from build123d import *

# Parameters (mm, degrees)
SKETCH1_W           = 8.5
SKETCH1_H           = 3.65
BOSS_EXTRUDE1_DEPTH = 1
SKETCH2_W           = 2.5
SKETCH2_H           = 2.05
BOSS_EXTRUDE2_DEPTH = 3
SKETCH3_W           = 4
SKETCH3_H           = 3.65
SKETCH3_W_2         = 3
BOSS_EXTRUDE3_DEPTH = 2.2
SKETCH4_W           = 8.5
SKETCH4_H           = 1
BOSS_EXTRUDE4_DEPTH = 1


with BuildPart() as part:
    # Sketch1 → Boss-Extrude1 (new body)
    with BuildSketch(Plane.XY):
        Rectangle(SKETCH1_W, SKETCH1_H)
    extrude(amount=BOSS_EXTRUDE1_DEPTH)

    # Sketch2 → Boss-Extrude2 (add)
    with BuildSketch(Plane.XY.offset(1)):
        Rectangle(SKETCH2_W, SKETCH2_H)
    extrude(amount=BOSS_EXTRUDE2_DEPTH)

    # Sketch3 → Boss-Extrude3 (add)
    with BuildSketch(Plane(origin=(0, 0, 0), x_dir=(-1, 0, 0), z_dir=(0, 0, -1))):
        with Locations((2.25, 0)):
            Rectangle(SKETCH3_W, SKETCH3_H)
        with Locations((-2.75, 0)):
            Rectangle(SKETCH3_W_2, SKETCH3_H)
    extrude(amount=BOSS_EXTRUDE3_DEPTH)

    # Sketch4 → Boss-Extrude4 (add)
    with BuildSketch(Plane(origin=(0, 1.825, 0), x_dir=(1, 0, 0), z_dir=(0, 1, 0))):
        with Locations((0, -0.5)):
            Rectangle(SKETCH4_W, SKETCH4_H)
    extrude(amount=BOSS_EXTRUDE4_DEPTH)


solid = part.part
Geometry check sheet. Reference: the model listing, model coordinates, mm. A direction names the side the tool comes from. Coordinates: 2 decimals unless noted, no trailing zeros. Order: outer loops, then holes, each group sorted by start corner. A loop starts at its lowest first (then second) coordinate and runs counter-clockwise, first axis right, second up. Notation, with made-up numbers: M 70.5,-31.75 L 82.5,-31.75 A13 ccw 82.5,-16.75 Z; hole C 28,65.25 d1. An arc over 180 degrees is marked long. Use CSV: the item, a comma, the result in double quotes.
Item 1: Cross-section at C-C on y = 0.7. Record the cut outline in (x, z), then the cut area to 3 significant figures.
Returned:
outline,"M -4.25,-2.2 L -0.25,-2.2 L -0.25,0 L 1.25,0 L 1.25,-2.2 L 4.25,-2.2 L 4.25,1 L 1.25,1 L 1.25,4 L -1.25,4 L -1.25,1 L -4.25,1 Z"
area,"31.4 mm2"
Item 2: Cross-section at B-B on x = -0.5. Record the cut outline in (y, z) (3 decimals).
Returned:
outline,"M -1.825,-2.2 L 1.825,-2.2 L 1.825,0 L 2.825,0 L 2.825,1 L 1.025,1 L 1.025,4 L -1.025,4 L -1.025,1 L -1.825,1 Z"
Item 3: Mould release check, pull along X, two halves, no side actions. Record for faces 4 (the flat face through (1.25, 0, -1)), 5 (the flat face through (0, 2, 0)), 6 (the flat face through (4.25, 0, -1)), 7 (the flat face through (0, 2, 1)): pulls with the +X half, pulls with the -X half, needs draft (parallel to the pull), parting line crosses it, or undercut.
Returned:
face 4,"undercut"
face 5,"undercut"
face 6,"pulls with the +X half"
face 7,"needs draft"
Item 4: Cross-section at D-D on x = 0.5. Record the cut outline in (y, z) (3 decimals), then the cut area to 3 significant figures.
Returned:
outline,"M -1.825,0 L 2.825,0 L 2.825,1 L 1.025,1 L 1.025,4 L -1.025,4 L -1.025,1 L -1.825,1 Z"
area,"10.8 mm2"
Item 5: Gauge pin test, flat ends, axial feed: pin 1 Ø0.7 at (x, z) = (2.5, -1) entering from +Y (3 decimals); pin 2 Ø1.5 at (x, y) = (2.5, 1.5) entering from +Z; pin 3 Ø1.6 at (y, z) = (-0.5, 2) entering from -X. Record the tip position at first contact, or that the pin passes through.
Returned:
pin 1,"stops at y = 1.825"
pin 2,"stops at z = 1"
pin 3,"stops at x = -1.25"
Item 6: Thickness scan on line 1 along X through (y, z) = (1.7, -1.5); line 2 along Z through (x, y) = (1.75, 0.35); line 3 along Y through (x, z) = (1.75, -1.5) (3 decimals). Record the ranges inside material, lowest first.
Returned:
line 1,"x = -4.25 to -0.25, 1.25 to 4.25"
line 2,"z = -2.2 to 1"
line 3,"y = -1.825 to 1.825"
Item 7: Tool access check on faces 1 (the flat face through (-0.25, 0, -1)), 2 (the flat face through (-1.25, 0, 2)), 3 (the flat face through (1.25, 0, 2)). Record the directions out of +Z, -Z, +X, -X, +Y, -Y that give a thin tool (end or side, any length) a straight path to the whole face; none if there is none.
Returned:
face 1,"-Z, +Y, -Y"
face 2,"+Z, -X, +Y, -Y"
face 3,"+Z, +X, +Y, -Y"
Item 8: Cross-section at A-A on z = -1.5. Record the cut outline in (x, y) (3 decimals), then the cut area to 4 significant figures.
Returned:
outline,"M -4.25,-1.825 L -0.25,-1.825 L -0.25,1.825 L -4.25,1.825 Z; M 1.25,-1.825 L 4.25,-1.825 L 4.25,1.825 L 1.25,1.825 Z"
area,"25.55 mm2"
